Input: part model. Units: mm. Frame: model coordinates. Face numbers are marked on the shaded views. A direction names the side the tool comes from. Coordinates: 2 decimals unless noted, no trailing zeros. Write each loop counter-clockwise with the first axis right and the second up, starting at its lowest first coordinate (ties: lowest second). Pieces come first, ordered by that corner, then holes. Notation, with made-up numbers: (11, 49.5) -> (38, 49.5) arc R28 cw to (38, 69.5) -> close; hole circle Ø4 at (80.25, -19). An arc over 180 degrees is marked (long way). One line per question, with ' | ' between items. Start each with the question number.
```python
from build123d import *

# Parameters (mm, degrees)
SKETCH1_W                = 20
SKETCH1_H                = 20
BOSS_EXTRUDE1_DEPTH      = 30
FILLET1_R                = 1
CUT_EXTRUDE1_DEPTH       = 34.166247904
F_5_0_5_DIAMETER_HOLE1_D = 5
FILLET2_R                = 2
FILLET3_R                = 0.5
FILLET4_R                = 0.5
FILLET5_R                = 0.5


with BuildPart() as part:
    # Sketch1 → Boss-Extrude1 (new body)
    with BuildSketch(Plane(origin=(0, 0, 0), x_dir=(0, 0, -1), z_dir=(1, 0, 0))):
        Rectangle(SKETCH1_W, SKETCH1_H)
    extrude(amount=BOSS_EXTRUDE1_DEPTH)

    # Fillet1
    fillet1_edges = [part.edges().sort_by_distance(p)[0] for p in [
        (15, 10, 10),
        (15, 10, -10),
        (15, -10, -10),
        (15, -10, 10),
    ]]
    fillet(fillet1_edges, radius=FILLET1_R)

    # Sketch3 → Cut-Extrude1 (cut, through all)
    with BuildSketch(Plane.ZY):
        Polygon((-3.6, 10), (3.6, 10), (3.6, 9.5), (3.1, 9.5), (3.1, 8.2), (5.63, 8.2), (5.63, 6.619949494), (2.910050506, 3.9), (-2.910050506, 3.9), (-5.63, 6.619949494), (-5.63, 8.2), (-3.1, 8.2), (-3.1, 9.5), (-3.6, 9.5), align=None)
        Polygon((10, 3.6), (10, -3.6), (9.5, -3.6), (9.5, -3.1), (8.2, -3.1), (8.2, -5.63), (6.619949494, -5.63), (3.9, -2.910050506), (3.9, 2.910050506), (6.619949494, 5.63), (8.2, 5.63), (8.2, 3.1), (9.5, 3.1), (9.5, 3.6), align=None)
        Polygon((3.6, -10), (-3.6, -10), (-3.6, -9.5), (-3.1, -9.5), (-3.1, -8.2), (-5.63, -8.2), (-5.63, -6.619949494), (-2.910050506, -3.9), (2.910050506, -3.9), (5.63, -6.619949494), (5.63, -8.2), (3.1, -8.2), (3.1, -9.5), (3.6, -9.5), align=None)
        Polygon((-10, -3.6), (-10, 3.6), (-9.5, 3.6), (-9.5, 3.1), (-8.2, 3.1), (-8.2, 5.63), (-6.619949494, 5.63), (-3.9, 2.910050506), (-3.9, -2.910050506), (-6.619949494, -5.63), (-8.2, -5.63), (-8.2, -3.1), (-9.5, -3.1), (-9.5, -3.6), align=None)
    extrude(amount=-CUT_EXTRUDE1_DEPTH, mode=Mode.SUBTRACT)

    # Ø5.0 (5) Diameter Hole1 (through all)
    with Locations(Plane.ZY):
        with Locations((0, 0)):
            Hole(F_5_0_5_DIAMETER_HOLE1_D / 2)

    # Fillet2
    fillet2_edges = [part.edges().sort_by_distance(p)[0] for p in [
        (15, -3.9, -2.910050506),
        (15, -3.9, 2.910050506),
        (15, 2.910050506, -3.9),
        (15, -2.910050506, -3.9),
        (15, -2.910050506, 3.9),
        (15, 2.910050506, 3.9),
        (15, 3.9, 2.910050506),
        (15, 3.9, -2.910050506),
    ]]
    fillet(fillet2_edges, radius=FILLET2_R)

    # Fillet3
    fillet3_edges = [part.edges().sort_by_distance(p)[0] for p in [
        (15, 3.6, -10),
        (15, 3.1, -9.5),
        (15, 3.1, -8.2),
        (15, 5.63, -8.2),
        (15, 5.63, -6.619949494),
        (15, 3.6, 10),
        (15, 3.1, 9.5),
        (15, 3.1, 8.2),
        (15, 5.63, 8.2),
        (15, 5.63, 6.619949494),
        (15, 6.619949494, 5.63),
        (15, 8.2, 5.63),
        (15, 8.2, 3.1),
        (15, 9.5, 3.1),
        (15, 10, 3.6),
        (15, 9.5, -3.1),
        (15, 10, -3.6),
        (15, 8.2, -3.1),
        (15, 8.2, -5.63),
        (15, 6.619949494, -5.63),
    ]]
    fillet(fillet3_edges, radius=FILLET3_R - 0.0001)  # a hair under: the kernel refuses the full size

    # Fillet4
    fillet4_edges = [part.edges().sort_by_distance(p)[0] for p in [
        (15, -3.6, 10),
        (15, -3.1, 9.5),
        (15, -3.1, 8.2),
        (15, -5.63, 8.2),
        (15, -5.63, 6.619949494),
        (15, -6.619949494, 5.63),
        (15, -8.2, 5.63),
        (15, -8.2, 3.1),
        (15, -10, 3.6),
        (15, -9.5, 3.1),
        (15, -10, -3.6),
        (15, -9.5, -3.1),
        (15, -8.2, -3.1),
        (15, -8.2, -5.63),
        (15, -6.619949494, -5.63),
        (15, -5.63, -6.619949494),
        (15, -5.63, -8.2),
        (15, -3.1, -8.2),
        (15, -3.1, -9.5),
        (15, -3.6, -10),
    ]]
    fillet(fillet4_edges, radius=FILLET4_R - 0.0001)  # a hair under: the kernel refuses the full size

    # Fillet5
    fillet5_edges = [part.edges().sort_by_distance(p)[0] for p in [
        (15, 3.6, 9.5),
        (15, 9.5, 3.6),
        (15, 9.5, -3.6),
        (15, 3.6, -9.5),
        (15, -3.6, 9.5),
        (15, -9.5, 3.6),
        (15, -9.5, -3.6),
        (15, -3.6, -9.5),
    ]]
    fillet(fillet5_edges, radius=FILLET5_R)


solid = part.part
```
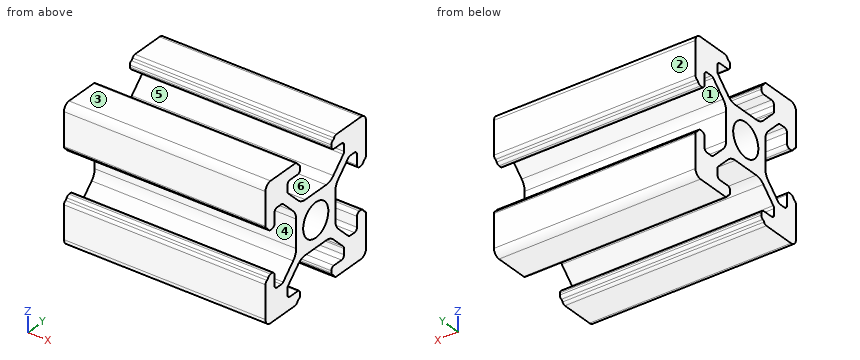
1) Section A-A, the plane z = 0. Return loops of the section in (x, y), then the cut area to 3 significant figures.
2) Access query for the marked faces 4, 5 and 6. Directions: +Z, -Z, +X, -X, +Y, -Y. A direction counts if a zero-diameter tool reaches every point of the face in a straight line with its end or side. Return the directions, or none.
3) Ray query, line 1 (Y direction, x = 14.5, z = 0); line 2 (Z direction, x = 25, y = -7); line 3 (Y direction, x = 18, z = 4.25). Return the intervals inside material, ascending.
4) First-contact query: P1, Ø1.2, axis at x = 17.5, z = 0, coming from the -Y side; P2, Ø3.5, axis at x = 11.5, y = 0, coming from the +Z side; P3, Ø1, axis at x = 23.5, z = 3, coming from the +Y side. Flat tips, straight axial feed; report the tip coordinate or a pass-through.
5) Pull-direction query (Y, two-part tool) for the marked faces 1, 2 and 3; classes: released by +Y, released by -Y, zero draft, split by the parting line, or undercut.
Answer block:
1) outline: (0, -3.9) -> (30, -3.9) -> (30, -2.5) -> (0, -2.5) -> close; (0, 2.5) -> (30, 2.5) -> (30, 3.9) -> (0, 3.9) -> close | area: 84.0 mm2
2) face 4: +X, -X, -Y | face 5: +X, -X | face 6: +Z, +X, -X
3) line 1: y = -3.9 to -2.5, 2.5 to 3.9 | line 2: z = -10 to -5.63, 5.63 to 10 | line 3: y = -10 to -8.2, -5.24 to -3.21, 3.21 to 5.24, 8.2 to 10
4) P1: stops at y = -3.9 | P2: stops at z = 3.9 | P3: stops at y = 9.52
5) face 1: undercut | face 2: released by +Y | face 3: zero draft
